from build123d import *

# Parameters (mm, degrees)
F1_DEPTH      = 2355.85
F2_W          = 68.2625
F2_H          = 19.05
F3_DEPTH      = 21.1863303725
F3_DEPTH_BACK = 16.9156696275


with BuildPart() as f1:
    # F0 (on Top) → F1 (new body)
    with BuildSketch(Plane.XY):
        Polygon((-2.1353303725, -12.5172607846), (-2.1353303725, 36.6952392154), (-21.1853303725, 36.6952392154), (-21.1853303725, -80.7797607846), (16.9146696275, -80.7797607846), (16.9146696275, -12.5172607846), align=None)
    extrude(amount=F1_DEPTH)

    # F2 (on Right) → F3 (cut, two sides)
    with BuildSketch(Plane.YZ) as f3_sk:
        with Locations((-46.6485107846, 2346.325)):
            Rectangle(F2_W, F2_H)
    extrude(amount=-F3_DEPTH, mode=Mode.SUBTRACT)
    extrude(f3_sk.sketch, amount=F3_DEPTH_BACK, mode=Mode.SUBTRACT)


solid = f1.part
Read the model definition and answer for the solid it produces. Units are mm, in the model's axes. A direction names the side the tool comes from. Give positions to 0.01 mm unless a question says otherwise; leave off trailing zeros. Write each loop counter-clockwise with the first axis right and the second up, starting at its lowest first coordinate (ties: lowest second). Pieces come first, ordered by that corner, then holes. Notation, with made-up numbers: (43.5, 80.25) -> (50.5, 80.25) arc R26 ccw to (50.5, 104.25) -> close; hole circle Ø6 at (19, 88). An arc over 180 degrees is marked (long way). Answer as a JSON object with one key per item and string values. Group by question number.
1) Each of these flat-tipped pins is pushed along its axis until it touches: P1, Ø11.5, axis at x = 6.5, y = -34.5, coming from the +Z side; P2, Ø8, axis at x = -8, y = -59, coming from the -Z side; P3, Ø24.5, axis at y = 2.5, z = 1048, coming from the +X side; P4, Ø5, axis at x = 7, z = 1433, coming from the +Y side. Where does it stop, or does it pass through?
2) Consider L1, parallel to Y at x = 3.5, z = 2013; L2, parallel to Z at x = -18, y = -31; L3, parallel to X at y = 2.5, z = 404. Determine where each line is inside the solid, lowest interval first. Write a range as from..to.
3) Find section A-A (z = 1723.5). Write down the section's boundary in (x, y), and give its area (3 significant figures).
4) Find section B-B (x = 8). Write down the section's boundary in (y, z).
5) A tool of negligible diameter and unlimited length cuts with its end or side. For faces 1 (the flat face through (-2, -47, 2336.8)), 2 (the flat face through (-2, -80.78, 1152)), 3 (the flat face through (-2.135, 12, 1161)), from which of +Z, -Z, +X, -X, +Y, -Y can it reach the whole face along a straight path? Write none if from no direction.
Values follow:
{
 "1": {"P1": "stops at z = 2336.8", "P2": "stops at z = 0", "P3": "stops at x = -2.14", "P4": "stops at y = -12.52"},
 "2": {"L1": "y = -80.78..-12.52", "L2": "z = 0..2336.8", "L3": "x = -21.19..-2.14"},
 "3": {"outline": "(-21.19, -80.78) -> (16.91, -80.78) -> (16.91, -12.52) -> (-2.14, -12.52) -> (-2.14, 36.7) -> (-21.19, 36.7) -> close", "area": "3,540 mm2"},
 "4": {"outline": "(-80.78, 0) -> (-12.52, 0) -> (-12.52, 2336.8) -> (-80.78, 2336.8) -> close"},
 "5": {"face 1": "+Z, +X, -X, -Y", "face 2": "+Z, -Z, +X, -X, -Y", "face 3": "+Z, -Z, +X, +Y"}
}
